from build123d import *

# Parameters (mm, degrees)
F1_W     = 50.8
F1_H     = 25.4
F1_R     = 4.8652202412
F2_DEPTH = 3.175


# Not quite as in the source:
# - a variable given as a bare number and used for a length is read in inches; the dataset says mm whatever the document's units were


with BuildPart() as f2:
    # F1 (on Right) → F2 (new body)
    with BuildSketch(Plane.YZ):
        Polygon((63.5, 7.14375), (-63.5, 7.14375), (-63.5, -7.14375), (12.7, -7.14375), (63.5, -7.14375), align=None)
        with Locations((38.1, -19.84375)):
            Rectangle(F1_W, F1_H)
        with Locations((19.9129190296, -13.6523451656)):
            Circle(F1_R, mode=Mode.SUBTRACT)
    extrude(amount=-F2_DEPTH)


solid = f2.part
Input: part model. Units: mm. Frame: model coordinates. A direction names the side the tool comes from. Coordinates: 2 decimals unless noted, no trailing zeros. Order: outer loops, then holes, each group sorted by start corner. A loop starts at its lowest first (then second) coordinate and runs counter-clockwise, first axis right, second up. Notation, with made-up numbers: M 17.25,-9 L 29.25,-9 A18 ccw 29.25,12 Z; hole C 39,3 d6. An arc over 180 degrees is marked long. Answer in a Markdown table with one row per item.
(1) Access query for faces 4 (the flat face through (-2, 1, 7.144)), 5 (the flat face through (-2, -26, -7.144)). Directions: +Z, -Z, +X, -X, +Y, -Y. A direction counts if a zero-diameter tool reaches every point of the face in a straight line with its end or side. Return the directions, or none.
Numbers:
| item | result |
|---|---|
| face 4 | +Z, +X, -X, +Y, -Y |
| face 5 | -Z, +X, -X, -Y |
(2) Section query A-A, the plane z = -29. Output: boundary loops of the cut face in (x, y) (3 decimals).
Numbers:
| item | result |
|---|---|
| outline | M -3.175,12.7 L 0,12.7 L 0,63.5 L -3.175,63.5 Z |
(3) Section query B-B, the plane x = -2.15. Output: boundary loops of the cut face in (y, z).
Numbers:
| item | result |
|---|---|
| outline | M -63.5,-7.14 L 12.7,-7.14 L 12.7,-32.54 L 63.5,-32.54 L 63.5,7.14 L -63.5,7.14 Z; hole C 19.91,-13.65 d9.73 |
(4) Material intervals for line 1 (Z direction, x = -2.2, y = 5.5); line 2 (Y direction, x = -2.4, z = -28); line 3 (Y direction, x = -1.35, z = -9.5), sorted ascending. Write a range as [from, to].
Numbers:
| item | result |
|---|---|
| line 1 | z = [-7.14, 7.14] |
| line 2 | y = [12.7, 63.5] |
| line 3 | y = [12.7, 17.38], [22.45, 63.5] |
(5) Section query C-C, the plane y = -55. Output: boundary loops of the cut face in (x, z) (3 decimals).
Numbers:
| item | result |
|---|---|
| outline | M -3.175,-7.144 L 0,-7.144 L 0,7.144 L -3.175,7.144 Z |
(6) Contact query for flat-ended pins moving along their axis: pin 1 Ø6 at (y, z) = (47.5, -0.5) entering from +X; pin 2 Ø1.6 at (x, y) = (-1.5, -21.5) entering from -Z. Output: stop coordinate, or through.
Numbers:
| item | result |
|---|---|
| pin 1 | stops at x = 0 |
| pin 2 | stops at z = -7.14 |
(7) Draft query along Y for faces 1 (the cylindrical face through (-1.565, 18.858, -18.402)), 2 (the flat face through (-2, -63.5, 0)), 3 (the flat face through (0, 13, -8)). Return one class per face: pulls with the +Y half, pulls with the -Y half, needs draft (parallel to the pull), parting line crosses it, or undercut.
Numbers:
| item | result |
|---|---|
| face 1 | undercut |
| face 2 | pulls with the -Y half |
| face 3 | needs draft |
